```python
from build123d import *

# Parameters (mm, degrees)
SKETCH1_R           = 2
BOSS_EXTRUDE1_DEPTH = 15
BOSS_EXTRUDE2_START = -35
SKETCH2_R           = 2
BOSS_EXTRUDE2_DEPTH = 35
SKETCH4_R           = 2
CUT_EXTRUDE1_DEPTH  = 10


with BuildPart() as part:
    # Sketch1 → Boss-Extrude1 (new body)
    with BuildSketch(Plane.XY):
        Polygon((130, -41.026010691), (130, -3.026010691), (124.226790646, 6.973481233), (76.026141267, 6.973481233), (72, 0), (-72, 0), (-76.026141267, 6.973481233), (-124.226790646, 6.973481233), (-130, -3.026010691), (-130, -41.026010691), (-120, -58.346518767), (120, -58.346518767), align=None)
        with Locations((-120, -7.026518767)):
            Circle(SKETCH1_R, mode=Mode.SUBTRACT)
        with Locations((-96.75, -7.026518767)):
            Circle(SKETCH1_R, mode=Mode.SUBTRACT)
        with Locations((-96.75, -30.276518767)):
            Circle(SKETCH1_R, mode=Mode.SUBTRACT)
        with Locations((-120, -30.276518767)):
            Circle(SKETCH1_R, mode=Mode.SUBTRACT)
        with Locations((120, -7.026518767)):
            Circle(SKETCH1_R, mode=Mode.SUBTRACT)
        with Locations((120, -30.276518767)):
            Circle(SKETCH1_R, mode=Mode.SUBTRACT)
        with Locations((96.75, -7.026518767)):
            Circle(SKETCH1_R, mode=Mode.SUBTRACT)
        with Locations((96.75, -30.276518767)):
            Circle(SKETCH1_R, mode=Mode.SUBTRACT)
        with Locations((0, -48.346518767)):
            Circle(SKETCH1_R, mode=Mode.SUBTRACT)
        with Locations((0, -22.346518767)):
            Circle(SKETCH1_R, mode=Mode.SUBTRACT)
    extrude(amount=BOSS_EXTRUDE1_DEPTH)

    # Sketch2 → Boss-Extrude2 (add)
    with BuildSketch(Plane.XY.offset(15).offset(BOSS_EXTRUDE2_START)):
        Polygon((-125.773502692, -48.346518767), (-120, -58.346518767), (120, -58.346518767), (125.773502692, -48.346518767), (30, -48.346518767), (30, -8.346518767), (-30, -8.346518767), (-30, -48.346518767), align=None)
        with Locations((0, -48.346518767)):
            Circle(SKETCH2_R, mode=Mode.SUBTRACT)
        with Locations((0, -22.346518767)):
            Circle(SKETCH2_R, mode=Mode.SUBTRACT)
    extrude(amount=BOSS_EXTRUDE2_DEPTH)

    # Sketch4 → Cut-Extrude1 (cut)
    with BuildSketch(Plane.XZ.offset(58.346518767)):
        with Locations((-72, -2.5)):
            Circle(SKETCH4_R)
        with Locations((-42, -2.5)):
            Circle(SKETCH4_R)
        with Locations(Location((42, -2.5, 0), (0, 0, 180))):
            Circle(SKETCH4_R)
        with Locations(Location((72, -2.5, 0), (0, 0, 180))):
            Circle(SKETCH4_R)
    extrude(amount=-CUT_EXTRUDE1_DEPTH, mode=Mode.SUBTRACT)


solid = part.part
```
The listing builds one solid part. Answer for the finished solid, in the listing's coordinates (mm). A direction names the side the tool comes from. Give positions to 0.01 mm unless a question says otherwise; leave off trailing zeros. Write each loop counter-clockwise with the first axis right and the second up, starting at its lowest first coordinate (ties: lowest second). Pieces come first, ordered by that corner, then holes. Notation, with made-up numbers: (31.5, -14) - (79.5, -14) arc R30 cw to (79.5, 16) - close; hole circle Ø7 at (-37.75, 0). An arc over 180 degrees is marked (long way). Use one line per item in the form item = value. Start each with the question number.
1) Flat-ended cylindrical pins translate along their axes: pin 1 Ø6.5 at (x, y) = (-120, -7.03) entering from -Z; pin 2 Ø1.5 at (y, z) = (-36, -2.5) entering from -X; pin 3 Ø16.5 at (x, z) = (5.5, 7) entering from +Y. Find the tip coordinate at first contact, or state that the pin passes through.
2) The mould has two halves that part along X. Classify faces 1 (the face through (-2, -25, 15)), 2 (the face through (130, -22, 7)), 3 (the face through (-127.1, 2, 7.4)), 4 (the face through (74.041, 3.536, 7.395)): pulls with the +X half, pulls with the -X half, needs draft (parallel to the pull), parting line crosses it, or undercut.
3) Find section A-A on z = -7. Determine the outline of the cut face in (x, y).
4) Consider line 1 along Y through (x, z) = (0, -1.5); line 2 along Y through (x, z) = (120, 7); line 3 along Z through (x, y) = (72, -56). Determine where each line is inside the solid, lowest interval first. Write a range as from..to.
5) Find section B-B on y = -44. Determine the outline of the cut face in (x, z).
6) A tool of negligible diameter and unlimited length cuts with its end or side. For faces 5 (the face through (1, 0, 7)), 6 (the face through (0, -8.347, -10)), 7 (the face through (-30, -28, -10)), 8 (the face through (30, -29, -10)), from which of +Z, -Z, +X, -X, +Y, -Y can it reach the whole face along a straight path? Write none if from no direction.
Geometry results:
q1.pin_1 = 0
q1.pin_2 = -30
q1.pin_3 = 0
q2.face_1 = needs draft
q2.face_2 = pulls with the +X half
q2.face_3 = pulls with the -X half
q2.face_4 = undercut
q3.outline = (-125.77, -48.35) - (-120, -58.35) - (120, -58.35) - (125.77, -48.35) - (30, -48.35) - (30, -8.35) - (-30, -8.35) - (-30, -48.35) - close; hole circle Ø4 at (0, -48.35); hole circle Ø4 at (0, -22.35)
q4.line_1 = -58.35..-50.35, -46.35..-24.35, -20.35..-8.35
q4.line_2 = -58.35..-32.28, -28.28..-9.03, -5.03..6.97
q4.line_3 = -20..-4.5, -0.5..15
q5.outline = (-128.28, 0) - (-30, 0) - (-30, -20) - (30, -20) - (30, 0) - (128.28, 0) - (128.28, 15) - (-128.28, 15) - close
q6.face_5 = +Z, -Z, +Y
q6.face_6 = -Z, +X, -X, +Y
q6.face_7 = -Z, -X, +Y
q6.face_8 = -Z, +X, +Y
